from build123d import *

# Parameters (mm, degrees)
PAD008_DEPTH            = 1.5
FILLET010_R             = 20
FILLET011_R             = 5
BODY009_PLACEMENT_ANGLE = 90


with BuildPart() as part:
    # Sketch013 → Pad008 (new body, symmetric)
    with BuildSketch(Plane.YZ):
        Polygon((27, -2.5), (61.9, -27.4), (61.9, 12.6), (27, 47.5), align=None)
    extrude(amount=PAD008_DEPTH, both=True)

    # Fillet010
    fillet010_edges = [part.edges().sort_by_distance(p)[0] for p in [
        (0, 61.9, 12.6),
    ]]
    fillet(fillet010_edges, radius=FILLET010_R)

    # Fillet011
    fillet011_edges = [part.edges().sort_by_distance(p)[0] for p in [
        (0, 27, -2.5),
    ]]
    fillet(fillet011_edges, radius=FILLET011_R)


with BuildPart() as part_1:
    # Body009 placement: moved
    add(part.part.moved(Location((30, 0, 0))).rotate(Axis((30, 0, 0), (0, 0, -1)), BODY009_PLACEMENT_ANGLE))


solid = part_1.part
Verification items for the finished model (mm, model axes). Coordinates: 2 decimals unless noted, no trailing zeros. Loops run counter-clockwise (first coordinate to the right, second up) from the corner with the lowest first, then second, coordinate; pieces in that order, holes last. Notation, with made-up numbers: (-29.75, -36) -> (-17.75, -36) arc R16 ccw to (-17.75, -31) -> close; hole circle Ø4 at (-9, 11.5). An arc over 180 degrees is marked (long way). Write each question's results on one line, items separated by ' | '.
Item 1: Section check C-C, the plane x = 69. Enter the section's corners in (y, z).
Found:
outline: (-1.5, -11.06) -> (1.5, -11.06) -> (1.5, 35.5) -> (-1.5, 35.5) -> close
Item 2: Material ranges on L1, parallel to Z at x = 70.5, y = 0.95; L2, parallel to Z at x = 76, y = 1.15; L3, parallel to X at y = 0.35, z = 35, recorded low to high.
Found:
L1: z = -12.13 to 34 | L2: z = -16.06 to 28.5 | L3: x = 57 to 69.5
Item 3: Section check B-B, the plane z = 37. Enter the section's corners in (x, y), plus the area to 3 significant figures.
Found:
outline: (57, -1.5) -> (67.5, -1.5) -> (67.5, 1.5) -> (57, 1.5) -> close | area: 31.5 mm2
Item 4: Section check A-A, the plane y = -0.9. Enter the section's corners in (x, z).
Found:
outline: (57, 0.07) arc R5 ccw to (59.1, -4) -> (91.9, -27.4) -> (91.9, 4.32) arc R20 ccw to (86.04, 18.46) -> (57, 47.5) -> close
